from build123d import *

# Parameters (mm, degrees)
BOSS_EXTRUDE1_DEPTH = 15.24
SKETCH2_R           = 3.175
CUT_EXTRUDE1_DEPTH  = 15.24


with BuildPart() as part:
    # Sketch1 → Boss-Extrude1 (new body)
    with BuildSketch(Plane(origin=(0, 0, 0), x_dir=(1, 0, 0), z_dir=(0, 1, 0))):
        with BuildLine():
            Line((31.75, 101.6), (31.75, 107.95))
            ThreePointArc((31.75, 107.95), (9.299359697, 98.650640303), (0, 76.2))
            Line((0, 76.2), (0, 0))
            Line((0, 0), (6.35, 0))
            Line((6.35, 0), (6.35, 76.2))
            ThreePointArc((6.35, 76.2), (13.789487758, 94.160512242), (31.75, 101.6))
        make_face()
    extrude(amount=BOSS_EXTRUDE1_DEPTH)

    # Sketch2 → Cut-Extrude1 (cut)
    with BuildSketch(Plane(origin=(6.35, 0, 0), x_dir=(0, 0, -1), z_dir=(1, 0, 0))):
        with Locations((6.35, 7.62)):
            Circle(SKETCH2_R)
    extrude(amount=-CUT_EXTRUDE1_DEPTH, mode=Mode.SUBTRACT)


solid = part.part
Design review of the part built by this model. Coordinates are the model's own, in mm. A direction names the side the tool comes from. Give positions to 0.01 mm unless a question says otherwise; leave off trailing zeros. Write each loop counter-clockwise with the first axis right and the second up, starting at its lowest first coordinate (ties: lowest second). Pieces come first, ordered by that corner, then holes. Notation, with made-up numbers: M 33.25,17.5 L 89.25,17.5 A28 cw 89.25,50.5 Z; hole C 0.5,-40 d4. An arc over 180 degrees is marked long. Answer as a JSON object with one key per item and string values. Group by question number.
1) We need section A-A (z = -6.35). Give the boundary of the cut face in (x, y) (3 decimals), and give its area (3 significant figures).
2) Mouldability with a two-part tool opening along Z and no side actions: class faces 1 (the face through (9.55, 7.51, -98.9)), 2 (the face through (31.75, 8, -105)), 3 (the face through (3.22, 5.69, -3.83)) as released by +Z, released by -Z, zero draft, split by the parting line, or undercut.
3) Clearance check with flat-ended pins moving along their axes: pin 1 Ø6 at (y, z) = (12.5, -95) entering from -X; pin 2 Ø1 at (x, y) = (16.5, 10) entering from +Z; pin 3 Ø1 at (y, z) = (12, -83.5) entering from +X. State where each tip first meets the part, or that it passes through.
4) For line 1 along Y through (x, z) = (4, -6.35) (3 decimals); line 2 along Y through (x, z) = (4, -6); line 3 along X through (y, z) = (2.5, -44), list the stretches that pass through material, from the lowest coordinate up.
5) Tool access review of faces 4 (the face through (5, 15.24, -58)), 5 (the face through (6.35, 8, -38)): name each direction out of +Z, -Z, +X, -X, +Y, -Y from which nothing blocks a thin tool from reaching the whole face with its end or side.
6) We need section C-C (z = -18). Give the boundary of the cut face in (x, y), and give its area (3 significant figures).
7) We need section D-D (y = 13.75). Give the boundary of the cut face in (x, z), and give its area (3 significant figures).
8) We need section B-B (y = 7.62). Give the boundary of the cut face in (x, z) (3 decimals).
Answer key:
{
 "1": {"outline": "M 0,0 L 6.35,0 L 6.35,4.445 L 0,4.445 Z; M 0,10.795 L 6.35,10.795 L 6.35,15.24 L 0,15.24 Z", "area": "56.5 mm²"},
 "2": {"face 1": "released by -Z", "face 2": "zero draft", "face 3": "undercut"},
 "3": {"pin 1": "stops at x = 4.21", "pin 2": "stops at z = -96.13", "pin 3": "stops at x = 7.58"},
 "4": {"line 1": "y = 0 to 4.445, 10.795 to 15.24", "line 2": "y = 0 to 4.46, 10.78 to 15.24", "line 3": "x = 0 to 6.35"},
 "5": {"face 4": "+Z, -Z, +X, -X, +Y", "face 5": "+Z, +X, +Y, -Y"},
 "6": {"outline": "M 0,0 L 6.35,0 L 6.35,15.24 L 0,15.24 Z", "area": "96.8 mm²"},
 "7": {"outline": "M 0,-76.2 A31.75 ccw 31.75,-107.95 L 31.75,-101.6 A25.4 cw 6.35,-76.2 L 6.35,0 L 0,0 Z", "area": "769 mm²"},
 "8": {"outline": "M 0,-76.2 A31.75 ccw 31.75,-107.95 L 31.75,-101.6 A25.4 cw 6.35,-76.2 L 6.35,-9.525 L 0,-9.525 Z; M 0,-3.175 L 6.35,-3.175 L 6.35,0 L 0,0 Z"}
}
